Part model, mm, in its own coordinate system. A direction names the side the tool comes from. Round coordinates to 2 decimals unless told otherwise and drop trailing zeros. Loops run counter-clockwise (first coordinate to the right, second up) from the corner with the lowest first, then second, coordinate; pieces in that order, holes last. Notation, with made-up numbers: (78.25, 36) -> (92.25, 36) arc R14 cw to (92.25, 43) -> close; hole circle Ø2 at (78, 14.5). An arc over 180 degrees is marked (long way). Use a Markdown table: item, result. Add a question column.
Item 1: Probe line 1 (Z direction, x = 0, y = 4.25); line 2 (Z direction, x = 0, y = 14.5); line 3 (X direction, y = 13.75, z = -16). List the from-to ranges inside material, lowest first. Write a range as [from, to].
Item 2: Flat gauge pins, fed straight in: pin 1 (3 mm diameter, centred on x = 0, z = -16, fed in from -Y); pin 2 (3 mm diameter, centred on x = 0, z = 16, fed in from +Y); pin 3 (3 mm diameter, centred on x = 5.5, z = -6, fed in from +Y). Where does each tip first touch, or does it go through?
Item 3: Two-plate mould, pull along X, no slides. Class faces 4 (the face through (2, 19, -17)), 5 (the face through (-7.5, 7, 0)), 6 (the face through (0, 12, 16)): pulls with the +X half, pulls with the -X half, needs draft (parallel to the pull), parting line crosses it, or undercut.
Item 4: Cut at A-A, the plane y = 13.25. List the corners of the cut face in (x, z), plus the area to 3 significant figures.
Item 5: Cut at C-C, the plane x = 0. List the corners of the cut face in (y, z), plus the area to 3 significant figures.
Item 6: Cut at D-D, the plane y = 9.5. List the corners of the cut face in (x, z).
Item 7: Which spindle directions (+Z, -Z, +X, -X, +Y, -Y) get a long thin tool onto all of the face, cutting with end or side? Do faces 1 (the face through (0, 3, 14)), 2 (the face through (0, 12, -16)), 3 (the face through (0, 9, 22)). Say none if no direction does.
Item 8: Cut at B-B, the plane z = 16. List the corners of the cut face in (x, y).
Autodesk Inventor part; units mm, degrees
ref_plane "YZ Plane" through (0, 0, 0) normal (1, 0, 0) x (0, 1, 0)
ref_plane "XZ Plane" through (0, 0, 0) normal (0, 1, 0) x (-1, 0, 0)
ref_plane "XY Plane" through (0, 0, 0) normal (0, 0, 1) x (1, 0, 0)
sketch "Эскиз1" plane through (0, 0, 0) normal (0, 1, 0) x (-1, 0, 0)
  line L0 (7.5, 22) -> (-7.5, 22)
  line L1 (-7.5, 22) -> (-7.5, -22)
  line L2 (-7.5, -22) -> (7.5, -22)
  line L3 (7.5, -22) -> (7.5, 22)
  line L4 (-7.5, 22) -> (7.5, -22) construction
  line L5 (0, 22) -> (0, -22) construction
  circle A0 centre (0, 16) radius 2
  line L6 (7.5, 0) -> (-7.5, 0) construction
  circle A1 centre (0, -16) radius 2
  point P0 (0, 0)
  point P1 (0, 0)
  dimension "d0" = 15
  dimension "d1" = 44
  dimension "d2" = 16
  dimension "d3" = 4
extrude "Выдавливание1" add sketch "Эскиз1" along normal blind 19
sketch "Эскиз2" plane through (7.5, 0, 22) normal (1, 0, 0) x (0, 0, -1)
  line L0 (0, 19) -> (44, 19)
  circle A0 centre (22, 19) radius 10.15
  point P0 (22, 0)
  dimension "d6" = 20.3
extrude "Выдавливание2" cut sketch "Эскиз2" against normal through all
ref_plane "РабПлоскость1" through (0, 12, 0) normal (0, 1, 0) x (1, 0, 0)
sketch "Эскиз3" plane through (0, 12, 0) normal (0, 1, 0) x (1, 0, 0)
  circle A0 centre (0, 16) radius 2
  circle A1 centre (0, -16) radius 2
  point P0 (0, 0)
extrude "Выдавливание3" add sketch "Эскиз3" against normal blind 5
properties part number "motor_mount_UP"
A:
| question | item | result |
|---|---|---|
| 1 | line 1 | z = [-22, -18], [-14, 14], [18, 22] |
| 1 | line 2 | z = [-22, -18], [-14, -9.1], [9.1, 14], [18, 22] |
| 1 | line 3 | x = [-7.5, -2], [2, 7.5] |
| 2 | pin 1 | stops at y = 7 |
| 2 | pin 2 | stops at y = 12 |
| 2 | pin 3 | stops at y = 12.16 |
| 3 | face 4 | needs draft |
| 3 | face 5 | pulls with the -X half |
| 3 | face 6 | undercut |
| 4 | outline | (-7.5, -22) -> (7.5, -22) -> (7.5, -8.36) -> (-7.5, -8.36) -> close; (-7.5, 8.36) -> (7.5, 8.36) -> (7.5, 22) -> (-7.5, 22) -> close; hole circle Ø4 at (0, -16); hole circle Ø4 at (0, 16) |
| 4 | area | 384 mm^2 |
| 5 | outline | (0, -22) -> (19, -22) -> (19, -18) -> (12, -18) -> (12, -14) -> (19, -14) -> (19, -10.15) arc R10.15 cw to (19, 10.15) -> (19, 14) -> (12, 14) -> (12, 18) -> (19, 18) -> (19, 22) -> (0, 22) -> (0, 18) -> (7, 18) -> (7, 14) -> (0, 14) -> (0, -14) -> (7, -14) -> (7, -18) -> (0, -18) -> close |
| 5 | area | 562 mm^2 |
| 6 | outline | (-7.5, -22) -> (7.5, -22) -> (7.5, -3.57) -> (-7.5, -3.57) -> close; (-7.5, 3.57) -> (7.5, 3.57) -> (7.5, 22) -> (-7.5, 22) -> close |
| 7 | face 1 | -Y |
| 7 | face 2 | +Y |
| 7 | face 3 | +Z, +X, -X, +Y, -Y |
| 8 | outline | (-7.5, 0) -> (-2, 0) -> (-2, 7) -> (2, 7) -> (2, 0) -> (7.5, 0) -> (7.5, 19) -> (2, 19) -> (2, 12) -> (-2, 12) -> (-2, 19) -> (-7.5, 19) -> close |
